```python
from build123d import *

# Parameters (mm, degrees)
BOSS_EXTRUDE1_REACH      = 829.277
BOSS_EXTRUDE1_END_RADIUS = 100
SKETCH2_R                = 38
SKETCH2_R_2              = 36.8


with BuildPart() as part:
    # Sketch1 → Revolve1 (revolve)
    with BuildSketch(Plane.XY, mode=Mode.PRIVATE) as revolve1_sk:
        Polygon((-100, 703.251175147), (-38, 703.251175147), (-38, 785.358038718), (-36.8, 785.358038718), (-36.8, 631.007989766), (-38, 631.007989766), (-38, 702.051175147), (-98.8, 702.051175147), (-98.8, 553.388924947), (-27.011266135, 244.817440016), (-88.8, 244.817440016), (-88.8, 1.2), (0, 1.2), (0, 0), (-90, 0), (-90, 246.017440016), (-28.522491796, 246.017440016), (-100, 553.251175147), align=None)
    revolve(revolve1_sk.sketch.rotate(Axis((0, 0, 0), (0, 1, 0)), 270), axis=Axis((0, 0, 0), (0, 1, 0)))

    # Boss-Extrude1: up to this cylinder (the profile starts outside it)
    boss_extrude1_end = Plane(origin=(0, 663.787131, 0), z_dir=(0, -1, 0)) * Cylinder(BOSS_EXTRUDE1_END_RADIUS, 1859.554, mode=Mode.PRIVATE)
    # Sketch2 → Boss-Extrude1 (add, up to the surface)
    with BuildSketch(Plane(origin=(140, 0, 0), x_dir=(0, 0, -1), z_dir=(1, 0, 0)), mode=Mode.PRIVATE) as boss_extrude1_sk1:
        with Locations((61.278662137, 663.787130772)):
            Circle(SKETCH2_R)
        with Locations((61.278662137, 663.787130772)):
            Circle(SKETCH2_R_2, mode=Mode.SUBTRACT)
    boss_extrude1_tool1 = extrude(boss_extrude1_sk1.sketch, amount=-BOSS_EXTRUDE1_REACH, mode=Mode.PRIVATE) - boss_extrude1_end
    add(boss_extrude1_tool1.solids().sort_by_distance((140, 663.787131, -24.353464))[0])


solid = part.part
```
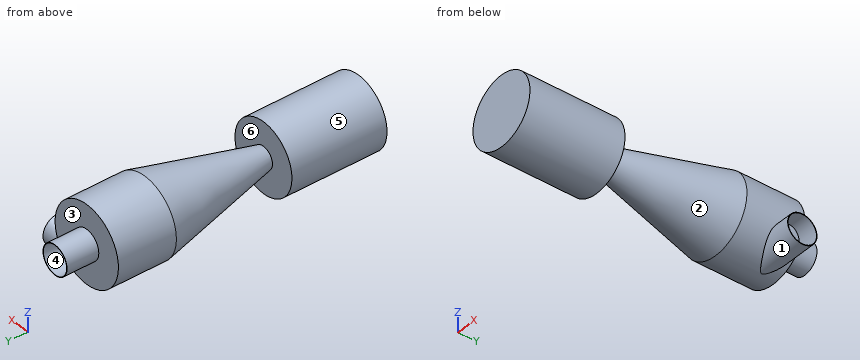
Read the model definition and answer for the solid it produces. Units are mm, in the model's axes. Face numbers are marked on the shaded views. A direction names the side the tool comes from. Give positions to 0.01 mm unless a question says otherwise; leave off trailing zeros. Loops run counter-clockwise (first coordinate to the right, second up) from the corner with the lowest first, then second, coordinate; pieces in that order, holes last.
Item 1: Each of these flat-tipped pins is pushed along its axis until it touches: pin 1 Ø2 at (x, y) = (86.5, 560) entering from +Z; pin 2 Ø2 at (x, z) = (-57.5, -65) entering from +Y; pin 3 Ø2 at (x, y) = (19, 668.5) entering from +Z. Where does it stop, or does it pass through?
Item 2: The mould has two halves that part along Z. Classify the marked faces 4, 5 and 6: released by +Z, released by -Z, zero draft, split by the parting line, or undercut.
Item 3: The part is cut by section D-D (x = 75.5). Give the number of separate pieces and of enclosed holes in the cut face, and give its area (3 significant figures).
Item 4: For the marked faces 1, 2 and 3, determine the directions among +Z, -Z, +X, -X, +Y, -Y from which every point of the face is accessible in a straight line to the end or side of a thin tool.
Item 5: Find the intervals of material crossed by line 1 along X through (y, z) = (69, 0); line 2 along Z through (x, y) = (3, 617); line 3 along Y through (x, z) = (7, -5), in increasing order.
Item 6: The part is cut by section A-A (y = 182.5). Write down the section's boundary in (x, z), and give its area (3 significant figures).
Taken from the geometry:
1. pin 1: stops at z = 51.86
1. pin 2: stops at y = 703.25
1. pin 3: stops at z = 98.37
2. face 4: undercut
2. face 5: split by the parting line
2. face 6: zero draft
3. separate pieces: 2
3. enclosed holes: 3
3. area: 2,850 mm2
4. face 1: +X
4. face 2: none
4. face 3: +Y
5. line 1: x = -90 to -88.8, 88.8 to 90
5. line 2: z = -99.95 to -98.75, 98.75 to 99.95
5. line 3: y = 0 to 1.2
6. outline: circle Ø180 at (0, 0); hole circle Ø177.6 at (0, 0)
6. area: 674 mm2
